Build history of the part. All positions in model axes, mm. Face numbers are marked on the shaded views. A direction names the side the tool comes from. Round coordinates to 2 decimals unless told otherwise and drop trailing zeros. Write each loop counter-clockwise with the first axis right and the second up, starting at its lowest first coordinate (ties: lowest second). Pieces come first, ordered by that corner, then holes.
Item 1: Wall check: probe 1 along Y at (x, z) = (0, 25); probe 2 along Z at (x, y) = (10, 20.5). Give the ranges that are in metal, low to high.
Item 2: Band-saw the part on D-D, the plane x = 24. Write the cut outline in (y, z), then the cut area to 3 significant figures.
Item 3: Band-saw the part on C-C, the plane z = 25. Write the cut outline in (x, y).
Item 4: Drop flat-ended pins along their axis: pin 1 Ø12 at (x, y) = (-68.5, 58.5) entering from +Z; pin 2 Ø4 at (x, y) = (-22.5, -47) entering from -Z; pin 3 Ø7 at (y, z) = (-12.5, 44) entering from -X; pin 4 Ø5 at (y, z) = (-10.5, 49) entering from +X. Give the stop position or say it passes through.
Item 5: 3-axis set-ups, long thin cutter, end or side, ignore diameter. For the marked faces 1 and 2: which of +Z, -Z, +X, -X, +Y, -Y reach the whole face in a straight line?
Item 6: Band-saw the part on B-B, the plane z = 44. Write the cut outline in (x, y), then the cut area to 3 significant figures.
Item 7: Band-saw the part on A-A, the plane y = 0. Write the cut outline in (x, z), then the cut area to 3 significant figures.
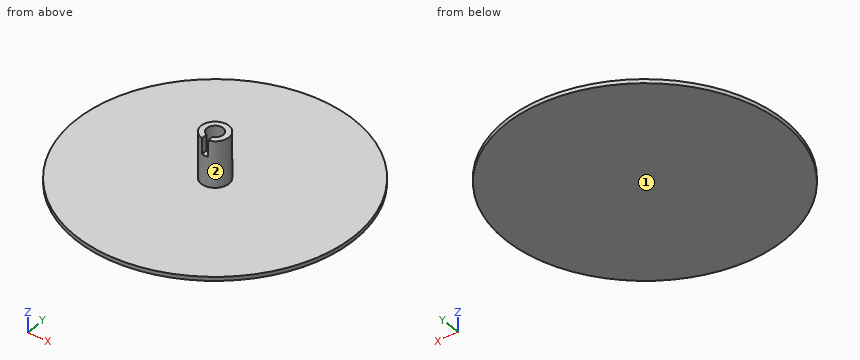
```python
from build123d import *

# Parameters (mm, degrees)
SCHIZZO1_R                   = 150
ESTRUSIONE_ESTRUSIONE1_DEPTH = 4.3
SCHIZZO2_R                   = 15
SCHIZZO2_R_2                 = 8.8
ESTRUSIONE_ESTRUSIONE2_DEPTH = 49.6
TAGLIO_ESTRUSIONE1_START     = -17.25
TAGLIO_ESTRUSIONE1_DEPTH     = 17.25


with BuildPart() as part:
    # Schizzo1 → Estrusione-Estrusione1 (new body)
    with BuildSketch(Plane.XY):
        Circle(SCHIZZO1_R)
    extrude(amount=ESTRUSIONE_ESTRUSIONE1_DEPTH)

    # Schizzo2 → Estrusione-Estrusione2 (add)
    with BuildSketch(Plane.XY.offset(4.3)):
        with Locations(Location((0, 0, 0), (0, 0, 180))):
            Circle(SCHIZZO2_R)
        with Locations(Location((0, 0, 0), (0, 0, 180))):
            Circle(SCHIZZO2_R_2, mode=Mode.SUBTRACT)
    extrude(amount=ESTRUSIONE_ESTRUSIONE2_DEPTH)

    # Schizzo3 → Taglio-Estrusione1 (cut)
    with BuildSketch(Plane.XY.offset(53.9).offset(TAGLIO_ESTRUSIONE1_START)):
        with BuildLine():
            Line((0, -15), (0, -8.8))
            ThreePointArc((0, -8.8), (-1.654505223, -8.643067307), (-3.25, -8.17786647))
            Line((-3.25, -8.17786647), (-3.25, -14.643684646))
            ThreePointArc((-3.25, -14.643684646), (-1.63473703, -14.910655078), (0, -15))
        make_face()
        with BuildLine():
            ThreePointArc((3.25, -8.17786647), (1.654505223, -8.643067307), (0, -8.8))
            Line((0, -8.8), (0, -15))
            ThreePointArc((0, -15), (1.63473703, -14.910655078), (3.25, -14.643684646))
            Line((3.25, -14.643684646), (3.25, -8.17786647))
        make_face()
    extrude(amount=TAGLIO_ESTRUSIONE1_DEPTH, mode=Mode.SUBTRACT)


solid = part.part
```
Results:
1. probe 1: y = -15 to -8.8, 8.8 to 15
1. probe 2: z = 0 to 4.3
2. outline: (-148.07, 0) - (148.07, 0) - (148.07, 4.3) - (-148.07, 4.3) - close
2. area: 1,270 mm2
3. outline: circle Ø30 at (0, 0); hole circle Ø17.6 at (0, 0)
4. pin 1: stops at z = 4.3
4. pin 2: stops at z = 0
4. pin 3: stops at x = -12
4. pin 4: stops at x = 12.69
5. face 1: -Z, +X, -X, +Y, -Y
5. face 2: +Z
6. outline: (-3.25, -14.64) - (-3.25, -8.18) arc R8.8 cw (long way) to (3.25, -8.18) - (3.25, -14.64) arc R15 ccw (long way) to start
6. area: 423 mm2
7. outline: (-150, 0) - (150, 0) - (150, 4.3) - (15, 4.3) - (15, 53.9) - (8.8, 53.9) - (8.8, 4.3) - (-8.8, 4.3) - (-8.8, 53.9) - (-15, 53.9) - (-15, 4.3) - (-150, 4.3) - close
7. area: 1,910 mm2
